```python
from build123d import *

# Parameters (mm, degrees)
F0_W     = 13.1206735969
F0_H     = 5.7628303766
F0_W_2   = 9.6076056361
F0_H_2   = 23.9247754216
F0_W_3   = 1.4953166246
F1_DEPTH = 25.4


with BuildPart() as f1:
    # F0 (on Front) → F1 (new body)
    with BuildSketch(Plane.XZ):
        Polygon((20.9109149873, 23.9247754216), (53.1037151814, 23.9247754216), (53.1037151814, 42.7394804328), (-51.2902662158, 34.7721107152), (-51.2902662158, 23.9247754216), align=None)
        Polygon((53.1037151814, 42.7394804328), (53.1037151814, 23.9247754216), (66.2243887782, 5.7628303766), (66.2243887782, 0), (85.0230753422, 0), (85.0230753422, 45.1755724388), align=None)
        Polygon((20.1173499505, 0), (20.9109149873, 23.9247754216), (-51.2902662158, 23.9247754216), (-51.2902662158, 0), align=None)
        Polygon((26.4795012772, 5.7628303766), (20.9109149873, 23.9247754216), (20.1173499505, 0), (26.4795012772, 0), align=None)
        with Locations((59.6640519798, 2.8814151883)):
            Rectangle(F0_W, F0_H)
        Polygon((53.1037151814, 57.1449995041), (53.1037151814, 42.7394804328), (85.0230753422, 45.1755724388), (85.0230753422, 57.1449995041), align=None)
        with Locations((-56.0940690339, 11.9623877108)):
            Rectangle(F0_W_2, F0_H_2)
        Polygon((-60.8978718519, 23.9247754216), (-51.2902662158, 23.9247754216), (-51.2902662158, 34.7721107152), (-60.8978718519, 34.0388563151), align=None)
        Polygon((26.4795012772, 0), (20.1173499505, 0), (26.4795012772, -20.7501575351), align=None)
        Polygon((66.2243887782, 0), (53.1037151814, 0), (64.2842540453, -17.6818622185), (66.2243887782, -19.0556111635), align=None)
        Polygon((-60.8978718519, 34.0388563151), (-51.2902662158, 34.7721107152), (-51.2902662158, 63.3518993855), (-60.8978718519, 63.3518993855), align=None)
        with Locations((-61.6455301642, 11.9623877108)):
            Rectangle(F0_W_3, F0_H_2)
        Polygon((-62.3931884766, 23.9247754216), (-60.8978718519, 23.9247754216), (-60.8978718519, 34.0388563151), (-193.4195458889, 23.9247754216), align=None)
        Polygon((39.3123003569, 0), (26.4795012772, 0), (26.4795012772, -20.7501575351), (66.2243887782, -20.7501575351), (64.2842540453, -17.6818622185), align=None)
        Polygon((66.2243887782, -19.0556111635), (64.2842540453, -17.6818622185), (66.2243887782, -20.7501575351), align=None)
        Polygon((-62.3931884766, 0), (-62.3931884766, 23.9247754216), (-193.4195458889, 23.9247754216), (-193.4195458889, -80.2987962961), (-62.3931884766, -80.2987962961), align=None)
    extrude(amount=F1_DEPTH)


solid = f1.part
```
The model under review builds one solid part; all positions refer to its coordinate system, in mm. A direction names the side the tool comes from. Round coordinates to 2 decimals unless told otherwise and drop trailing zeros. Loops run counter-clockwise (first coordinate to the right, second up) from the corner with the lowest first, then second, coordinate; pieces in that order, holes last. Notation, with made-up numbers: (5, 12) - (42, 12) arc R26 cw to (42, 41) - close; hole circle Ø4 at (43, -14.5). An arc over 180 degrees is marked (long way). Write each question's results on one line, items separated by ' | '. Start each with the question number.
Q1. Take a section at D-D on x = -17. Give the boundary of the cut face in (y, z), plus the area to 3 significant figures.
Q2. Take a section at C-C on z = 13.5. Give the boundary of the cut face in (x, y), plus the area to 3 significant figures.
Q3. Draft analysis for pull direction Z (two halves, no side actions). For faces 1 (the flat face through (-62.393, -13, -41)), 2 (the flat face through (51.973, -12.522, -8.965)), 3 (the flat face through (-126.231, -12.522, 29.053)), 4 (the flat face through (60, -13, 5.763)), state which applies: pulls with the +Z half, pulls with the -Z half, needs draft (parallel to the pull), parting line crosses it, or undercut.
Q4. Take a section at B-B on x = 36.5. Give the boundary of the cut face in (y, z).
Q5. Wall thickness on line 1 along X through (y, z) = (-5.75, 4); line 2 along Z through (x, y) = (28.5, -4.75); line 3 along X through (y, z) = (-2.75, -54): over which ranges is each line inside the solid? List them lowest first. Write a range as [from, to].
Q6. Insertion check: P1, Ø12.5, axis at y = -13, z = -53, coming from the +X side; P2, Ø6, axis at x = -143, y = -6, coming from the +Z side; P3, Ø6, axis at x = 56.5, y = -7, coming from the +Z side (3 decimals). Each pin has a flat end and moves straight along its axis. Give the tip position at first contact, or say it passes through.
Q7. Tool access review of faces 5 (the flat face through (37, -13, 23.925)), 6 (the flat face through (-22, -13, 0)), 7 (the flat face through (53.104, -13, 50)), 8 (the flat face through (69, -13, 57.145)): name each direction out of +Z, -Z, +X, -X, +Y, -Y from which nothing blocks a thin tool from reaching the whole face with its end or side.
Q8. Take a section at A-A on y = -3.75. Give the boundary of the cut face in (x, z) (1 decimal).
Data:
1) outline: (-25.4, 0) - (0, 0) - (0, 37.39) - (-25.4, 37.39) - close | area: 950 mm²
2) outline: (-193.42, -25.4) - (24.11, -25.4) - (24.11, 0) - (-193.42, 0) - close; (60.63, -25.4) - (85.02, -25.4) - (85.02, 0) - (60.63, 0) - close | area: 6,140 mm²
3) face 1: needs draft | face 2: undercut | face 3: pulls with the +Z half | face 4: undercut
4) outline: (-25.4, -20.75) - (0, -20.75) - (0, 0) - (-25.4, 0) - close; (-25.4, 23.92) - (0, 23.92) - (0, 41.47) - (-25.4, 41.47) - close
5) line 1: x = [-193.42, 26.48], [53.1, 85.02] | line 2: z = [-20.75, 0], [23.92, 40.86] | line 3: x = [-193.42, -62.39]
6) P1: stops at x = -62.39 | P2: stops at z = 28 | P3: stops at z = 57.145
7) face 5: +Y, -Y | face 6: -Z, +Y, -Y | face 7: +Z, +Y, -Y | face 8: +Z, +X, +Y, -Y
8) outline: (-193.4, -80.3) - (-62.4, -80.3) - (-62.4, 0) - (20.1, 0) - (26.5, -20.8) - (66.2, -20.8) - (66.2, 0) - (85, 0) - (85, 57.1) - (53.1, 57.1) - (53.1, 42.7) - (-51.3, 34.8) - (-51.3, 63.4) - (-60.9, 63.4) - (-60.9, 34) - (-193.4, 23.9) - close; hole (20.9, 23.9) - (26.5, 5.8) - (26.5, 0) - (39.3, 0) - (64.3, -17.7) - (53.1, 0) - (53.1, 5.8) - (66.2, 5.8) - (53.1, 23.9) - close
